Answer from the drawing. Dimensions are ordinates in mm from the lowest x, y and z of the part. Coordinates: 2 decimals unless noted, no trailing zeros. Loops run counter-clockwise (first coordinate to the right, second up) from the corner with the lowest first, then second, coordinate; pieces in that order, holes last. Notation, with made-up numbers: M -8,50 L 38,50 A22 cw 38,74 Z; hole C 74.5,70.5 d10. An arc over 180 degrees is marked long. Put each result on its own line as item: value.
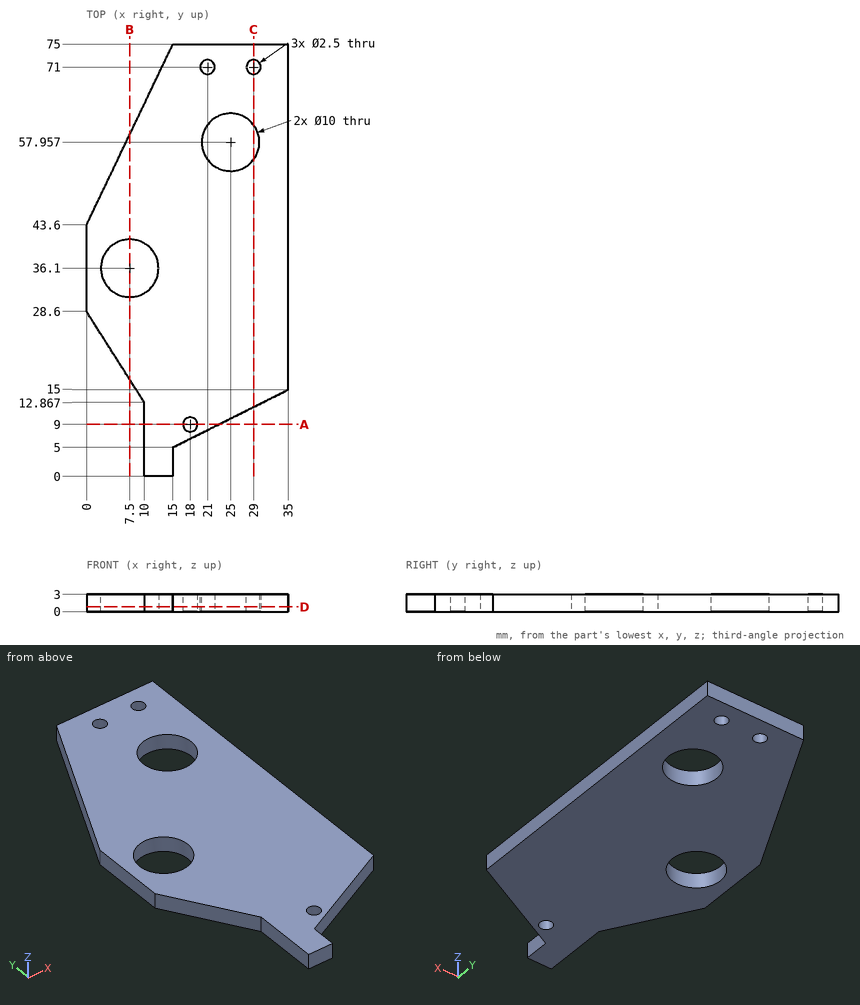
1) Find section A-A, the plane y = 9. Write down the section's boundary in (x, z).
Answer list:
outline: M 10,0 L 16.75,0 L 16.75,3 L 10,3 Z; M 19.25,0 L 23,0 L 23,3 L 19.25,3 Z
2) Straight lines are drawn through the part: line 1 (Y direction, x = 25, z = 2.2); line 2 (Y direction, x = 11.5, z = 1.2) (1 decimal); line 3 (X direction, y = 71, z = 1.6). For each, find the intervals that lie inside material, in ascending order. Write a range as [from, to].
Answer list:
line 1: y = [10, 52.96], [62.96, 75]
line 2: y = [0, 33.1], [39.1, 67.7]
line 3: x = [13.09, 19.75], [22.25, 27.75], [30.25, 35]
3) Find section D-D, the plane z = 0.8. Write down the section's boundary in (x, y), plus the area to 3 significant figures.
Answer list:
outline: M 0,28.6 L 10,12.87 L 10,0 L 15,0 L 15,5 L 35,15 L 35,75 L 15,75 L 0,43.6 Z; hole C 7.5,36.1 d10; hole C 18,9 d2.5; hole C 21,71 d2.5; hole C 25,57.96 d10; hole C 29,71 d2.5
area: 1,810 mm^2
4) Find section C-C, the plane x = 29. Write down the section's boundary in (y, z).
Answer list:
outline: M 12,0 L 54.96,0 L 54.96,3 L 12,3 Z; M 60.96,0 L 69.75,0 L 69.75,3 L 60.96,3 Z; M 72.25,0 L 75,0 L 75,3 L 72.25,3 Z
5) Given pin 1 Ø2 at (x, y) = (18, 9) entering from +Z, flat-ended and moving along its own axis, determine where the tip first touches the part or whether it passes through.
Answer list:
pin 1: passes through
6) Find section B-B, the plane x = 7.5. Write down the section's boundary in (y, z).
Answer list:
outline: M 16.8,0 L 31.1,0 L 31.1,3 L 16.8,3 Z; M 41.1,0 L 59.3,0 L 59.3,3 L 41.1,3 Z
